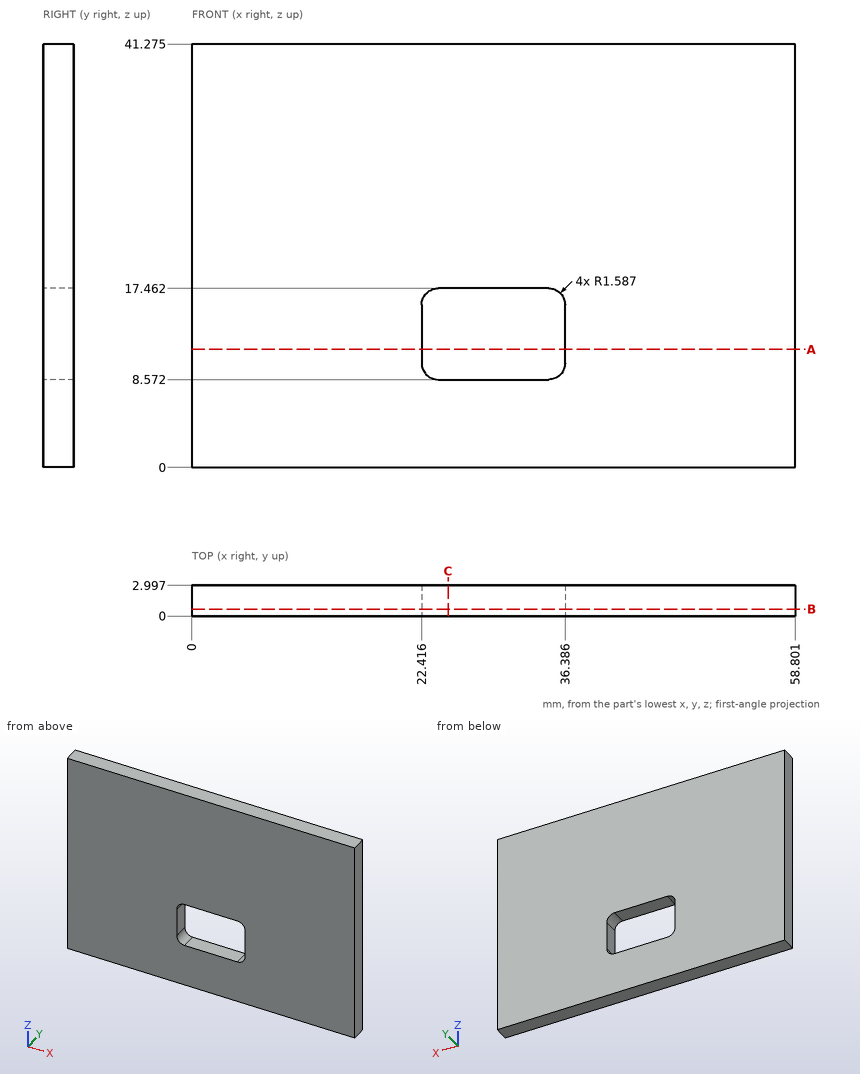
Could you check a few things on this drawing? It's one solid part, dimensions in mm from its lowest x, y, z. Give positions to 0.01 mm unless a question says otherwise; leave off trailing zeros. Write each loop counter-clockwise with the first axis right and the second up, starting at its lowest first coordinate (ties: lowest second). Pieces come first, ordered by that corner, then holes. Notation, with made-up numbers: (85, 88.5) -> (91, 88.5) arc R23 ccw to (91, 97.5) -> close; hole circle Ø2 at (0, 42). An arc over 180 degrees is marked (long way). Answer as CSV lines item,"result". Start each with the question number.
(1) If we section it at A-A, the plane z = 11.5: Write out the boundary of the cut face in (x, y) (1 decimal).
(2) Please list where these lines run through material, in increasing order: line 1 (X direction, y = 2.2, z = 10.5) (1 decimal); line 2 (Z direction, x = 34, y = 2.15) (1 decimal); line 3 (X direction, y = 0.1, z = 16.5) (1 decimal).
(3) I'm going to push a flat-ended pin straight in: pin 1 Ø1.5 at (y, z) = (2, 13) entering from -X. Where does the tip first touch, or does it pass through?
(4) If we section it at C-C, the plane x = 25: Write out the boundary of the cut face in (y, z) (1 decimal).
(5) If we section it at B-B, the plane y = 0.7: Write out the boundary of the cut face in (x, z) (1 decimal), and give its area (4 significant figures).
Answer list:
1,outline,"(0, 0) -> (22.4, 0) -> (22.4, 3) -> (0, 3) -> close; (36.4, 0) -> (58.8, 0) -> (58.8, 3) -> (36.4, 3) -> close"
2,line 1,"0 to 22.4, 36.4 to 58.8"
2,line 2,"0 to 8.6, 17.5 to 41.3"
2,line 3,"0 to 22.5, 36.3 to 58.8"
3,pin 1,"x = 0"
4,outline,"(0, 0) -> (3, 0) -> (3, 8.6) -> (0, 8.6) -> close; (0, 17.5) -> (3, 17.5) -> (3, 41.3) -> (0, 41.3) -> close"
5,outline,"(0, 0) -> (58.8, 0) -> (58.8, 41.3) -> (0, 41.3) -> close; hole (22.4, 10.2) arc R1.6 ccw to (24, 8.6) -> (34.8, 8.6) arc R1.6 ccw to (36.4, 10.2) -> (36.4, 15.9) arc R1.6 ccw to (34.8, 17.5) -> (24, 17.5) arc R1.6 ccw to (22.4, 15.9) -> close"
5,area,"2,305 mm^2"
